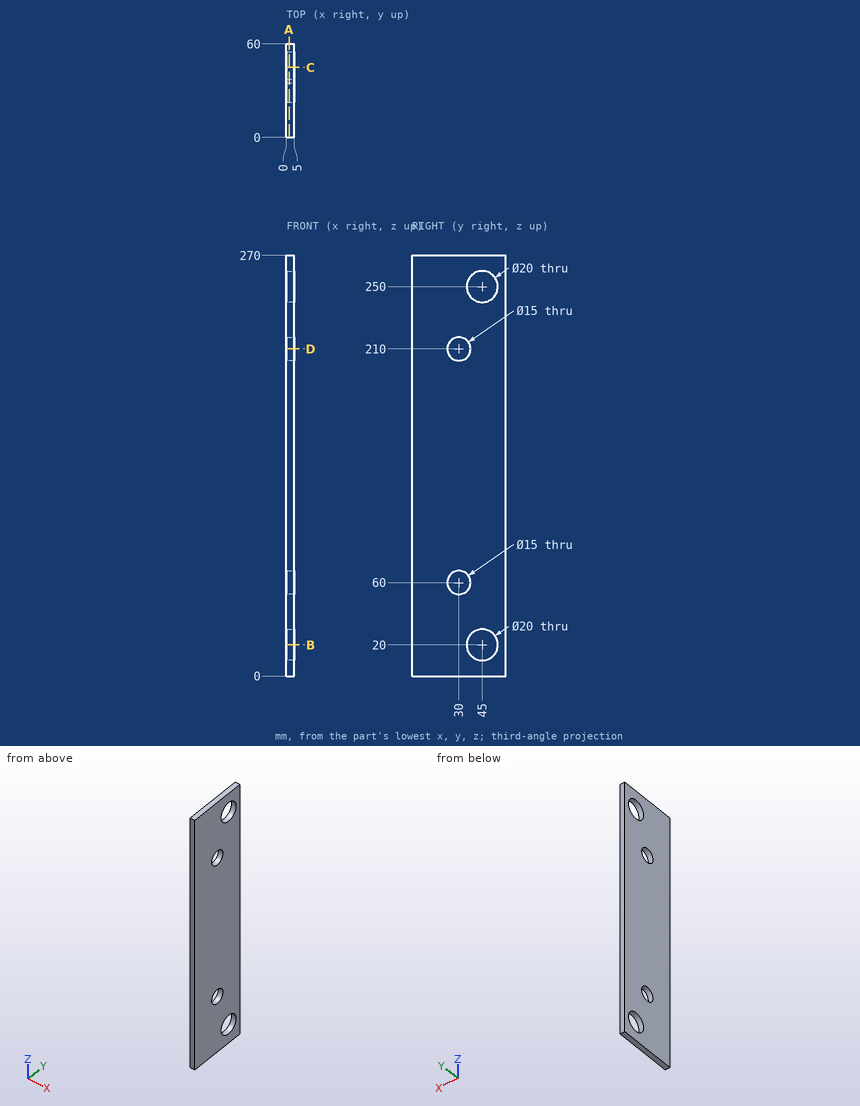
Here's the drawing with two shaded views (mm, measured from the low corner). I have some questions. Round coordinates to 2 decimals unless told otherwise and drop trailing zeros. Loops run counter-clockwise (first coordinate to the right, second up) from the corner with the lowest first, then second, coordinate; pieces in that order, holes last. Notation, with made-up numbers: M 72.5,72 L 77.5,72 A21 cw 77.5,103 Z; hole C 40,86.25 d8. An arc over 180 degrees is marked long. Answer as a JSON object with one key per item and string values. Group by question number.
Q1. Imagine slicing it at A-A, the plane x = 1.7. Please give me the cut outline in (y, z).
Q2. Imagine slicing it at D-D, the plane z = 210. Please give me the cut outline in (x, y).
Q3. Imagine slicing it at B-B, the plane z = 20. Please give me the cut outline in (x, y).
Q4. Imagine slicing it at C-C, the plane y = 45. Please give me the cut outline in (x, z).
Q5. Please list where these lines run through material, in increasing order: L1, parallel to Y at x = 3.15, z = 210; L2, parallel to Z at x = 0.4, y = 27; L3, parallel to Y at x = 2.5, z = 250.
Findings:
{
 "1": {"outline": "M 0,0 L 60,0 L 60,270 L 0,270 Z; hole C 30,60 d15; hole C 30,210 d15; hole C 45,20 d20; hole C 45,250 d20"},
 "2": {"outline": "M 0,0 L 5,0 L 5,22.5 L 0,22.5 Z; M 0,37.5 L 5,37.5 L 5,60 L 0,60 Z"},
 "3": {"outline": "M 0,0 L 5,0 L 5,35 L 0,35 Z; M 0,55 L 5,55 L 5,60 L 0,60 Z"},
 "4": {"outline": "M 0,0 L 5,0 L 5,10 L 0,10 Z; M 0,30 L 5,30 L 5,240 L 0,240 Z; M 0,260 L 5,260 L 5,270 L 0,270 Z"},
 "5": {"L1": "y = 0 to 22.5, 37.5 to 60", "L2": "z = 0 to 53.13, 66.87 to 203.13, 216.87 to 270", "L3": "y = 0 to 35, 55 to 60"}
}
